from build123d import *

# Parameters (mm, degrees)
CROQUIS1_W              = 35
CROQUIS1_H              = 35
SALIENTE_EXTRUIR1_DEPTH = 385
CROQUIS2_W              = 35
CROQUIS2_H              = 35
SALIENTE_EXTRUIR2_DEPTH = 235
CROQUIS3_R              = 15
CORTAR_EXTRUIR1_DEPTH   = 35


with BuildPart() as part:
    # Croquis1 → Saliente-Extruir1 (new body)
    with BuildSketch(Plane.XY):
        Rectangle(CROQUIS1_W, CROQUIS1_H)
    extrude(amount=SALIENTE_EXTRUIR1_DEPTH)

    # Croquis2 → Saliente-Extruir2 (add)
    with BuildSketch(Plane(origin=(0, 17.5, 0), x_dir=(1, 0, 0), z_dir=(0, 1, 0))):
        with Locations((0, -17.5)):
            Rectangle(CROQUIS2_W, CROQUIS2_H)
    extrude(amount=SALIENTE_EXTRUIR2_DEPTH)

    # Croquis3 → Cortar-Extruir1 (cut)
    with BuildSketch(Plane(origin=(0, 0, 0), x_dir=(-1, 0, 0), z_dir=(0, 0, -1))):
        with Locations((0, 207.5)):
            Circle(CROQUIS3_R)
    extrude(amount=-CORTAR_EXTRUIR1_DEPTH, mode=Mode.SUBTRACT)


solid = part.part
Read the model definition and answer for the solid it produces. Units are mm, in the model's axes. A direction names the side the tool comes from. Round coordinates to 2 decimals unless told otherwise and drop trailing zeros. Loops run counter-clockwise (first coordinate to the right, second up) from the corner with the lowest first, then second, coordinate; pieces in that order, holes last.
Q1. Section A-A on x = 0 is taken. Write down the section's boundary in (y, z).
Q2. Section B-B on y = 207.5 is taken. Write down the section's boundary in (x, z).
Q3. Which of the six approach directions +Z, -Z, +X, -X, +Y, -Y give full straight-line access (tool end or side, diameter ignored) to faces 1 (the face through (0, 17.5, 208)), 2 (the face through (0, 252.5, 17))?
Q4. Section C-C on z = 188.5 is taken. Write down the section's boundary in (x, y).
Q5. Each of these flat-tipped pins is pushed along its axis until it touches: pin 1 (5 mm diameter, centred on x = 8, y = 128.5, fed in from +Z); pin 2 (4 mm diameter, centred on x = 12.5, z = 60, fed in from +Y); pin 3 (12 mm diameter, centred on x = 8, y = 68, fed in from -Z). Where does it stop, or does it pass through?
Q6. Determine the mould class of faces 3 (the face through (0, 0, 385)), 4 (the face through (0, -17.5, 190)), 5 (the face through (3.252, 192.857, 17.255)) for opening direction Y: released by +Y, released by -Y, zero draft, split by the parting line, or undercut.
Q7. Consider probe 1 along Y at (x, z) = (0, 25); probe 2 along Z at (x, y) = (-10, 117.5); probe 3 along Y at (x, z) = (11, 64.5). Determine where each line is inside the solid, lowest interval first.
Output:
1. outline: (-17.5, 0) - (192.5, 0) - (192.5, 35) - (17.5, 35) - (17.5, 385) - (-17.5, 385) - close; (222.5, 0) - (252.5, 0) - (252.5, 35) - (222.5, 35) - close
2. outline: (-17.5, 0) - (-15, 0) - (-15, 35) - (-17.5, 35) - close; (15, 0) - (17.5, 0) - (17.5, 35) - (15, 35) - close
3. face 1: +Z, +X, -X, +Y
3. face 2: +Z, -Z, +X, -X, +Y
4. outline: (-17.5, -17.5) - (17.5, -17.5) - (17.5, 17.5) - (-17.5, 17.5) - close
5. pin 1: stops at z = 35
5. pin 2: stops at y = 17.5
5. pin 3: stops at z = 0
6. face 3: zero draft
6. face 4: released by -Y
6. face 5: undercut
7. probe 1: y = -17.5 to 192.5, 222.5 to 252.5
7. probe 2: z = 0 to 35
7. probe 3: y = -17.5 to 17.5
